For this review, use the dimensioned drawing (mm, ordinates from the lowest corner) and the shaded views. Give positions to 0.01 mm unless a question says otherwise; leave off trailing zeros. Order: outer loops, then holes, each group sorted by start corner. A loop starts at its lowest first (then second) coordinate and runs counter-clockwise, first axis right, second up. Notation, with made-up numbers: M 27,0.25 L 60,0.25 A24 ccw 60,38.25 Z; hole C 35,31 d10. An arc over 180 degrees is marked long. One line per question, with ' | ' between items. Start each with the question number.
1. We need section C-C on y = 120. Write out the cut boundary in (x, z).
2. Wall thickness on L1, parallel to Y at x = 10, z = 3.75; L2, parallel to Y at x = 163.5, z = 9: over which ranges is each line inside the solid? List them lowest first.
3. We need section B-B on y = 10. Write out the cut boundary in (x, z).
4. Insertion check: P1, Ø5, axis at x = 163, y = 120, coming from the +Z side; P2, Ø4, axis at x = 142, z = 6.5, coming from the -Y side. Each pin has a flat end and moves straight along its axis. Give the tip position at first contact, or say it passes through.
5. We need section D-D on x = 290. Write out the cut boundary in (y, z).
6. We need section A-A on x = 133. Write out the cut boundary in (y, z).
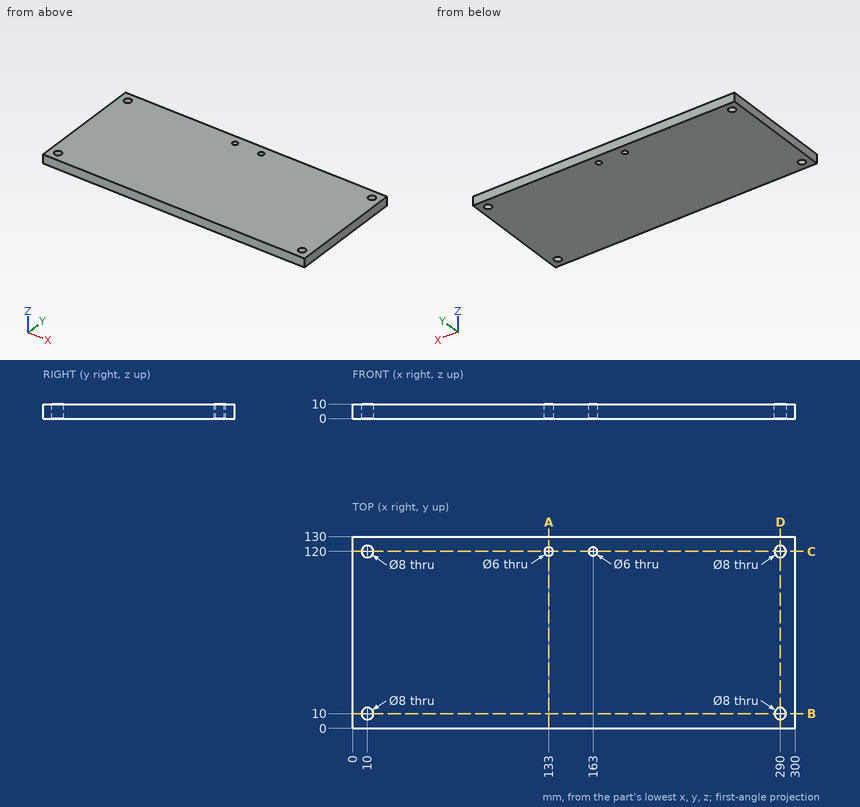
Entries:
1) outline: M 0,0 L 6,0 L 6,10 L 0,10 Z; M 14,0 L 130,0 L 130,10 L 14,10 Z; M 136,0 L 160,0 L 160,10 L 136,10 Z; M 166,0 L 286,0 L 286,10 L 166,10 Z; M 294,0 L 300,0 L 300,10 L 294,10 Z
2) L1: y = 0 to 6, 14 to 116, 124 to 130 | L2: y = 0 to 117.04, 122.96 to 130
3) outline: M 0,0 L 6,0 L 6,10 L 0,10 Z; M 14,0 L 286,0 L 286,10 L 14,10 Z; M 294,0 L 300,0 L 300,10 L 294,10 Z
4) P1: passes through | P2: stops at y = 0
5) outline: M 0,0 L 6,0 L 6,10 L 0,10 Z; M 14,0 L 116,0 L 116,10 L 14,10 Z; M 124,0 L 130,0 L 130,10 L 124,10 Z
6) outline: M 0,0 L 117,0 L 117,10 L 0,10 Z; M 123,0 L 130,0 L 130,10 L 123,10 Z
